```python
from build123d import *

# Parameters (mm, degrees)
SKETCH_1_W          = 11
SKETCH_1_H          = 5.45
EXTRUDE_1_DEPTH     = 44
SKETCH_3_R          = 1.5
CUT_EXTRUDE_2_DEPTH = 49.548944376


with BuildPart() as part:
    # 草图1 → 凸台-拉伸1 (new body)
    with BuildSketch(Plane.XY):
        with BuildLine():
            Line((2, -10), (7.5, -10))
            Line((7.5, -10), (7.5, 14))
            Line((7.5, 14), (-7.5, 14))
            Line((-7.5, 14), (-7.5, -10))
            Line((-7.5, -10), (-2, -10))
            Line((-2, -10), (-2, -3.521718331))
            ThreePointArc((-2, -3.521718331), (0, 4.05), (2, -3.521718331))
            Line((2, -3.521718331), (2, -10))
        make_face()
        with Locations((0, 9.275)):
            Rectangle(SKETCH_1_W, SKETCH_1_H, mode=Mode.SUBTRACT)
    extrude(amount=EXTRUDE_1_DEPTH)

    # 草图3 → 切除-拉伸2 (cut, through all)
    with BuildSketch(Plane.ZY.offset(7.5)):
        with Locations((7, -7)):
            Circle(SKETCH_3_R)
        with Locations((37, -7)):
            Circle(SKETCH_3_R)
        with Locations((22, 8)):
            Circle(SKETCH_3_R)
    extrude(amount=-CUT_EXTRUDE_2_DEPTH, mode=Mode.SUBTRACT)


solid = part.part
```
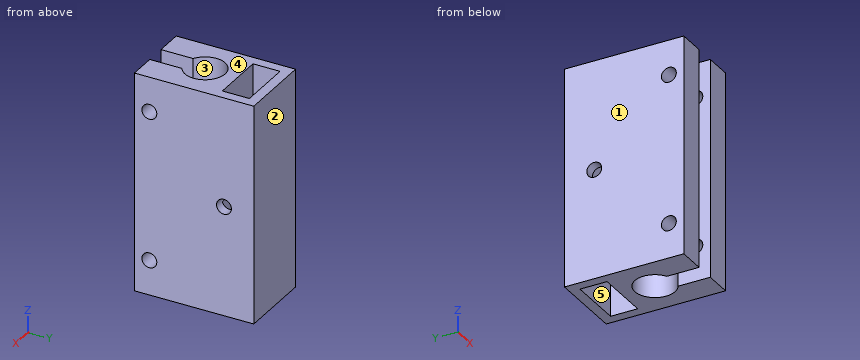
Could you check a few things on this model? Use its own coordinates, in mm. Face numbers are marked on the shaded views. A direction names the side the tool comes from. Coordinates: 2 decimals unless noted, no trailing zeros. Write each loop counter-clockwise with the first axis right and the second up, starting at its lowest first coordinate (ties: lowest second). Pieces come first, ordered by that corner, then holes. Notation, with made-up numbers: (5, 23.5) -> (41, 23.5) arc R21 ccw to (41, 42.5) -> close; hole circle Ø6 at (-23, 5.25). An arc over 180 degrees is marked (long way). One line per question, with ' | ' between items. Start each with the question number.
1. If we section it at C-C (y = -7): Please give me the cut outline in (x, z).
2. If we section it at D-D (y = 0): Please give me the cut outline in (x, z).
3. If we section it at B-B (x = 0): Please give me the cut outline in (y, z), and give its area (3 significant figures).
4. Please list where these lines run through material, in increasing order: line 1 along X through (y, z) = (-7.75, 34.5); line 2 along Y through (x, z) = (-0.25, 16.5); line 3 along X through (y, z) = (0, 30.5).
5. Thinking about a two-plate mould opening in Y: for the marked faces 1, 2 and 3, which applies, pulls with the +Y half, pulls with the -Y half, needs draft (parallel to the pull), parting line crosses it, or undercut?
6. Will this pin go through, and if not, where does the flat tip stop? P1, Ø4, axis at x = 1, z = 32, coming from the -Y side.
7. If we section it at A-A (z = 7): Please give me the cut outline in (x, y), and give its area (3 significant figures).
8. For the marked faces 4 and 5, which set-ups out of +Z, -Z, +X, -X, +Y, -Y let a thin tool reach every point of the face, with its end or its side?
Return value:
1) outline: (-7.5, 0) -> (-2, 0) -> (-2, 5.5) -> (-7.5, 5.5) -> close; (-7.5, 8.5) -> (-2, 8.5) -> (-2, 35.5) -> (-7.5, 35.5) -> close; (-7.5, 38.5) -> (-2, 38.5) -> (-2, 44) -> (-7.5, 44) -> close; (2, 0) -> (7.5, 0) -> (7.5, 5.5) -> (2, 5.5) -> close; (2, 8.5) -> (7.5, 8.5) -> (7.5, 35.5) -> (2, 35.5) -> close; (2, 38.5) -> (7.5, 38.5) -> (7.5, 44) -> (2, 44) -> close
2) outline: (-7.5, 0) -> (-4.05, 0) -> (-4.05, 44) -> (-7.5, 44) -> close; (4.05, 0) -> (7.5, 0) -> (7.5, 44) -> (4.05, 44) -> close
3) outline: (4.05, 0) -> (6.55, 0) -> (6.55, 21.62) arc R1.5 cw to (6.55, 22.38) -> (6.55, 44) -> (4.05, 44) -> close; (12, 0) -> (14, 0) -> (14, 44) -> (12, 44) -> close | area: 198 mm²
4) line 1: x = -7.5 to -2, 2 to 7.5 | line 2: y = 4.04 to 6.55, 12 to 14 | line 3: x = -7.5 to -4.05, 4.05 to 7.5
5) face 1: needs draft | face 2: pulls with the +Y half | face 3: undercut
6) P1: stops at y = -10
7) outline: (-7.5, -10) -> (-2, -10) -> (-2, -8.5) -> (-7.5, -8.5) -> close; (-7.5, -5.5) -> (-2, -5.5) -> (-2, -3.52) arc R4.05 cw (long way) to (2, -3.52) -> (2, -5.5) -> (7.5, -5.5) -> (7.5, 14) -> (-7.5, 14) -> close; (2, -10) -> (7.5, -10) -> (7.5, -8.5) -> (2, -8.5) -> close; hole (-5.5, 6.55) -> (5.5, 6.55) -> (5.5, 12) -> (-5.5, 12) -> close | area: 191 mm²
8) face 4: +Z, +X, -X, +Y, -Y | face 5: +Z, -Z
